```python
from build123d import *

# Parameters (mm, degrees)
F1_DEPTH = 3.45
F5_D     = 3.3


with BuildPart() as f1:
    # F0 (on Top) → F1 (new body)
    with BuildSketch(Plane.XY):
        Polygon((5, -2.8867513459), (5, 2.8867513459), (0, 5.7735026919), (-5, 2.8867513459), (-5, -2.8867513459), (0, -5.7735026919), align=None)
    extrude(amount=F1_DEPTH)

    # F2 (on Front) → F3 (revolve, cut)
    with BuildSketch(Plane.XZ):
        Polygon((6.9201928239, 3.45), (5, 3.45), (6.9201928239, 2.751106968), align=None)
    revolve(axis=Axis((0, 0, 1.725), (0, 0, 1)), mode=Mode.SUBTRACT)

    # F5 (through all)
    with Locations(Plane.XY.offset(3.45)):
        with Locations((0, 0)):
            Hole(F5_D / 2)


solid = f1.part
```
Input: part model. Units: mm. Frame: model coordinates. Give positions to 0.01 mm unless a question says otherwise; leave off trailing zeros. Loops run counter-clockwise (first coordinate to the right, second up) from the corner with the lowest first, then second, coordinate; pieces in that order, holes last.
1) Contact query for flat-ended pins moving along their axis: pin 1 (1.5 mm diameter, centred on x = 3.5, z = 1.5, fed in from +Y); pin 2 (2 mm diameter, centred on x = 0, y = 0, fed in from +Z); pin 3 (1.5 mm diameter, centred on x = -1.5, z = 1, fed in from -Y). Output: stop coordinate, or through.
A:
pin 1: stops at y = 4.19
pin 2: passes through
pin 3: stops at y = -5.34
2) Line query: L1, parallel to Y at x = 0.25, z = 0.4; L2, parallel to Y at x = -1.5, z = 2.5; L3, parallel to X at y = -4, z = 1.3. Output: solid intervals per line, ascending.
A:
L1: y = -5.63 to -1.63, 1.63 to 5.63
L2: y = -4.91 to -0.69, 0.69 to 4.91
L3: x = -3.07 to 3.07
3) Mould query, pull axis Z, two halves, no side actions, for faces 1 (the flat face through (-1.2, 1.4, 0)), 2 (the flat face through (2, 0, 3.45)), 3 (the flat face through (2.535, 4.31, 1.701)). Classes: released by +Z, released by -Z, zero draft, split by the parting line, or undercut.
A:
face 1: released by -Z
face 2: released by +Z
face 3: zero draft
4) Section query A-A on z = 0.65. Return the cut outline in (x, y), and give its area (3 significant figures).
A:
outline: (-5, -2.89) - (0, -5.77) - (5, -2.89) - (5, 2.89) - (0, 5.77) - (-5, 2.89) - close; hole circle Ø3.3 at (0, 0)
area: 78.0 mm2
